Read the model definition and answer for the solid it produces. Units are mm, in the model's axes. A direction names the side the tool comes from. Give positions to 0.01 mm unless a question says otherwise; leave off trailing zeros. Loops run counter-clockwise (first coordinate to the right, second up) from the corner with the lowest first, then second, coordinate; pieces in that order, holes last.
(1) Find section C-C, the plane x = 47. Write down the section's boundary in (y, z), then the cut area to 3 significant figures.
(2) Straight lines are drawn through the part: probe 1 along Y at (x, z) = (13.5, 190); probe 2 along Z at (x, y) = (35.5, 101.5). For each, find the intervals that lie inside material, in ascending order.
(3) Find section B-B, the plane z = 217.5. Write down the section's boundary in (x, y).
(4) Find section A-A, the plane y = 76. Write down the section's boundary in (x, z), then the cut area to 3 significant figures.
(5) Find section D-D, the plane x = 62. Write down the section's boundary in (y, z).
(6) Each of these flat-tipped pins is pushed along its axis until it touches: P1, Ø1.8, axis at x = 39.5, z = 181, coming from the +Y side; P2, Ø4, axis at y = 53.5, z = 181.5, coming from the -X side; P3, Ø0.8, axis at x = 45, z = 181, coming from the -Y side; P4, Ø2.5, axis at x = 43.46, y = 91.09, coming from the -Z side. Where does it stop, or does it pass through?
(7) Determine the mould class of faces 1 (the face through (52, 65, 181.644)), 2 (the face through (86.173, 65, 181)), 3 (the face through (42.99, 88.99, 180.83)) for opening direction X: pulls with the +X half, pulls with the -X half, needs draft (parallel to the pull), parting line crosses it, or undercut.
(8) Which of the six approach directions +Z, -Z, +X, -X, +Y, -Y give full straight-line access (tool end or side, diameter ignored) to faces 4 (the face through (24.45, 89.18, 180.83)), 5 (the face through (43, 132.181, 206))?
```python
from build123d import *

# Parameters (mm, degrees)
SKETCH1_R                    = 2.15265
SKETCH1_W                    = 20
SKETCH1_H                    = 30
BASE_FLANGE1_DEPTH           = 1.6002
SKETCHED_BEND1_OUTLINE_W     = 86.92285
SKETCHED_BEND1_OUTLINE_H     = 1.6002
SKETCHED_BEND1_DEPTH         = 180.344310973
SKETCHED_START               = 183.63
SKETCHED_BEND1_2_OUTLINE_W   = 86.92285
SKETCHED_BEND1_2_OUTLINE_H   = 1.6002
SKETCHED_BEND1_2_DEPTH       = 46.5
SKETCHED_START_2             = 181.496703893
SKETCHED_BEND1_3_OUTLINE_W   = 85.42285
SKETCHED_BEND1_3_OUTLINE_H   = 132.181185133
SKETCHED_BEND1_3_OUTLINE_R   = 2.15265
SKETCHED_BEND1_3_OUTLINE_W_2 = 20
SKETCHED_BEND1_3_OUTLINE_H_2 = 30
SKETCHED_BEND1_3_DEPTH       = 0.14770354
SKETCHED_START_3             = 182.965207433
SKETCHED_BEND1_4_OUTLINE_W   = 85.42285
SKETCHED_BEND1_4_OUTLINE_H   = 1.6002
SKETCHED_BEND1_4_DEPTH       = 0.664792567
SKETCHED_START_4             = 180.044207433
SKETCHED_BEND1_5_OUTLINE_W   = 85.42285
SKETCHED_BEND1_5_OUTLINE_H   = 132.181185133
SKETCHED_BEND1_5_OUTLINE_R   = 2.15265
SKETCHED_BEND1_5_OUTLINE_W_2 = 20
SKETCHED_BEND1_5_OUTLINE_H_2 = 30
SKETCHED_BEND1_5_DEPTH       = 2.921
SKETCHED_START_5             = 0.75
SKETCHED_BEND1_6_DEPTH       = 85.42285
SKETCHED_START_6             = 132.181185133
SKETCHED_BEND1_7_DEPTH       = 1.6002
SKETCHED_BEND1_8_DEPTH       = 85.42285


with BuildPart() as part:
    # Base-Flange1: sheet metal written as solids
    # Sketch1 → Base-Flange1 (new body)
    with BuildSketch(Plane(origin=(0, 0, 0), x_dir=(1, 0, 0), z_dir=(0, 1, 0))):
        with BuildLine():
            Line((0.75, -46.6), (0.75, -183.53))
            ThreePointArc((0.75, -183.53), (0.720710678, -183.600710678), (0.65, -183.63))
            Line((0.65, -183.63), (0, -183.63))
            Line((0, -183.63), (0, -230.13))
            Line((0, -230.13), (86.92285, -230.13))
            Line((86.92285, -230.13), (86.92285, -183.63))
            Line((86.92285, -183.63), (86.27285, -183.63))
            ThreePointArc((86.27285, -183.63), (86.202139322, -183.600710678), (86.17285, -183.53))
            Line((86.17285, -183.53), (86.17285, -46.6))
            ThreePointArc((86.17285, -46.6), (86.202139322, -46.529289322), (86.27285, -46.5))
            Line((86.27285, -46.5), (86.92285, -46.5))
            Line((86.92285, -46.5), (86.92285, 0))
            Line((86.92285, 0), (0, 0))
            Line((0, 0), (0, -46.5))
            Line((0, -46.5), (0.65, -46.5))
            ThreePointArc((0.65, -46.5), (0.720710678, -46.529289322), (0.75, -46.6))
        make_face()
        with Locations(Location((43.461425, -90.065, 0), (0, 0, 270))):
            Circle(SKETCH1_R, mode=Mode.SUBTRACT)
        with Locations(Location((43.461425, -140.065, 0), (0, 0, 270))):
            Circle(SKETCH1_R, mode=Mode.SUBTRACT)
        with Locations(Location((23.461425, -90.065, 0), (0, 0, 270))):
            Circle(SKETCH1_R, mode=Mode.SUBTRACT)
        with Locations(Location((23.461425, -140.065, 0), (0, 0, 270))):
            Circle(SKETCH1_R, mode=Mode.SUBTRACT)
        with Locations((41.461425, -115.065)):
            Rectangle(SKETCH1_W, SKETCH1_H, mode=Mode.SUBTRACT)
    extrude(amount=-BASE_FLANGE1_DEPTH)

    # Sketched Bend1: read off the stored shape, not the designer's step
    # Sketched Bend1 outline → Sketched Bend1 (cut)
    with BuildSketch(Plane.XY):
        with Locations((43.461425, -0.8001)):
            Rectangle(SKETCHED_BEND1_OUTLINE_W, SKETCHED_BEND1_OUTLINE_H)
    extrude(amount=SKETCHED_BEND1_DEPTH, mode=Mode.SUBTRACT)

    # Sketched Bend1 3 outline → Sketched Bend1 3 (add)
    with BuildSketch(Plane.XY.offset(SKETCHED_START_2)):
        with Locations((43.461425, 66.090592567)):
            Rectangle(SKETCHED_BEND1_3_OUTLINE_W, SKETCHED_BEND1_3_OUTLINE_H)
        with Locations((23.461425, 41.090592567)):
            Circle(SKETCHED_BEND1_3_OUTLINE_R, mode=Mode.SUBTRACT)
        with Locations((43.461425, 41.090592567)):
            Circle(SKETCHED_BEND1_3_OUTLINE_R, mode=Mode.SUBTRACT)
        with Locations((41.461425, 66.090592567)):
            Rectangle(SKETCHED_BEND1_3_OUTLINE_W_2, SKETCHED_BEND1_3_OUTLINE_H_2, mode=Mode.SUBTRACT)
        with Locations((23.461425, 91.090592567)):
            Circle(SKETCHED_BEND1_3_OUTLINE_R, mode=Mode.SUBTRACT)
        with Locations((43.461425, 91.090592567)):
            Circle(SKETCHED_BEND1_3_OUTLINE_R, mode=Mode.SUBTRACT)
    extrude(amount=SKETCHED_BEND1_3_DEPTH)



with BuildPart() as body_2:
    # Sketched Bend1 2 outline → Sketched Bend1 2 (new body)
    with BuildSketch(Plane.XY.offset(SKETCHED_START)):
        with Locations((43.461425, 132.981285133)):
            Rectangle(SKETCHED_BEND1_2_OUTLINE_W, SKETCHED_BEND1_2_OUTLINE_H)
    extrude(amount=SKETCHED_BEND1_2_DEPTH)

    # Sketched Bend1 4 outline → Sketched Bend1 4 (add)
    with BuildSketch(Plane.XY.offset(SKETCHED_START_3)):
        with Locations((43.461425, 132.981285133)):
            Rectangle(SKETCHED_BEND1_4_OUTLINE_W, SKETCHED_BEND1_4_OUTLINE_H)
    extrude(amount=SKETCHED_BEND1_4_DEPTH)


with BuildPart() as part_1:
    add(part.part)

    add(body_2.part)  # Sketched Bend1 5 merges body 2
    # Sketched Bend1 5 outline → Sketched Bend1 5 (add)
    with BuildSketch(Plane.XY.offset(SKETCHED_START_4)):
        with Locations((43.461425, 66.090592567)):
            Rectangle(SKETCHED_BEND1_5_OUTLINE_W, SKETCHED_BEND1_5_OUTLINE_H)
        with Locations((23.461425, 41.090592567)):
            Circle(SKETCHED_BEND1_5_OUTLINE_R, mode=Mode.SUBTRACT)
        with Locations((43.461425, 41.090592567)):
            Circle(SKETCHED_BEND1_5_OUTLINE_R, mode=Mode.SUBTRACT)
        with Locations((41.461425, 66.090592567)):
            Rectangle(SKETCHED_BEND1_5_OUTLINE_W_2, SKETCHED_BEND1_5_OUTLINE_H_2, mode=Mode.SUBTRACT)
        with Locations((23.461425, 91.090592567)):
            Circle(SKETCHED_BEND1_5_OUTLINE_R, mode=Mode.SUBTRACT)
        with Locations((43.461425, 91.090592567)):
            Circle(SKETCHED_BEND1_5_OUTLINE_R, mode=Mode.SUBTRACT)
    extrude(amount=SKETCHED_BEND1_5_DEPTH)

    # Sketched Bend1 6 outline → Sketched Bend1 6 (add)
    with BuildSketch(Plane.YZ.offset(SKETCHED_START_5)):
        with BuildLine():
            Line((133.781385133, 182.965207433), (132.181185133, 182.965207433))
            Line((132.181185133, 182.965207433), (132.181185133, 180.359880513))
            ThreePointArc((132.181185133, 180.359880513), (133.349390737, 181.436452352), (133.781385133, 182.965207433))
        make_face()
    extrude(amount=SKETCHED_BEND1_6_DEPTH)

    # Sketched Bend1 7 outline → Sketched Bend1 7 (add)
    with BuildSketch(Plane(origin=(0, 0, 0), x_dir=(1, 0, 0), z_dir=(0, 1, 0)).offset(SKETCHED_START_6)):
        with BuildLine():
            Line((0.75, -183.63), (0.75, -183.53))
            ThreePointArc((0.75, -183.53), (0.720710678, -183.600710678), (0.65, -183.63))
            Line((0.65, -183.63), (0.75, -183.63))
        make_face()
        with BuildLine():
            ThreePointArc((86.27285, -183.63), (86.202139322, -183.600710678), (86.17285, -183.53))
            Line((86.17285, -183.53), (86.17285, -183.63))
            Line((86.17285, -183.63), (86.27285, -183.63))
        make_face()
    extrude(amount=SKETCHED_BEND1_7_DEPTH)

    # Sketched Bend1 8 outline → Sketched Bend1 8 (cut)
    with BuildSketch(Plane.YZ.offset(SKETCHED_START_5)):
        with BuildLine():
            ThreePointArc((130.860385133, 181.644407433), (131.79433177, 182.031260796), (132.181185133, 182.965207433))
            Line((132.181185133, 182.965207433), (0, 182.965207433))
            ThreePointArc((0, 182.965207433), (0.386853363, 182.031260796), (1.3208, 181.644407433))
            Line((1.3208, 181.644407433), (130.860385133, 181.644407433))
        make_face()
        with BuildLine():
            Line((132.181185133, 180.044207433), (132.181185133, 180.359880513))
            ThreePointArc((132.181185133, 180.359880513), (131.539384789, 180.124221607), (130.860385133, 180.044207433))
            Line((130.860385133, 180.044207433), (132.181185133, 180.044207433))
        make_face()
        with BuildLine():
            Line((0, 180.04420738), (1.3208, 180.044207433))
            ThreePointArc((1.3208, 180.044207433), (-0.744658907, 180.899748526), (-1.6002, 182.965207433))
            Line((-1.6002, 182.965207433), (-1.600200001, 185))
            Line((-1.600200001, 185), (-3, 185))
            Line((-3, 185), (-3, 180.344310973))
            Line((-3, 180.344310973), (0, 180.344310973))
            Line((0, 180.344310973), (0, 180.04420738))
        make_face()
    extrude(amount=SKETCHED_BEND1_8_DEPTH, mode=Mode.SUBTRACT)


solid = part_1.part
```
Entries:
1. outline: (-1.6, 182.97) arc R2.92 ccw to (1.32, 180.04) - (51.09, 180.04) - (51.09, 181.64) - (1.32, 181.64) arc R1.32 cw to (0, 182.97) - (0, 230.13) - (-1.6, 230.13) - close; (81.09, 180.04) - (130.86, 180.04) arc R2.92 ccw to (133.78, 182.97) - (133.78, 230.13) - (132.18, 230.13) - (132.18, 182.97) arc R1.32 cw to (130.86, 181.64) - (81.09, 181.64) - close
1. area: 321 mm2
2. probe 1: y = -1.6 to 0, 132.18 to 133.78
2. probe 2: z = 180.04 to 181.64
3. outline: (0, -1.6) - (86.92, -1.6) - (86.92, 0) - (0, 0) - close; (0, 132.18) - (86.92, 132.18) - (86.92, 133.78) - (0, 133.78) - close
4. outline: (0.75, 180.04) - (31.46, 180.04) - (31.46, 181.64) - (0.75, 181.64) - close; (51.46, 180.04) - (86.17, 180.04) - (86.17, 181.64) - (51.46, 181.64) - close
4. area: 105 mm2
5. outline: (-1.6, 182.97) arc R2.92 ccw to (1.32, 180.04) - (130.86, 180.04) arc R2.92 ccw to (133.78, 182.97) - (133.78, 230.13) - (132.18, 230.13) - (132.18, 182.97) arc R1.32 cw to (130.86, 181.64) - (1.32, 181.64) arc R1.32 cw to (0, 182.97) - (0, 230.13) - (-1.6, 230.13) - close
6. P1: stops at y = 133.58
6. P2: stops at x = 0.75
6. P3: stops at y = -1.15
6. P4: passes through
7. face 1: needs draft
7. face 2: pulls with the +X half
7. face 3: undercut
8. face 4: +Z, -Z
8. face 5: +Z, +X, -X
